Input: part model. Units: mm. Frame: model coordinates. Face numbers are marked on the shaded views. A direction names the side the tool comes from. Round coordinates to 2 decimals unless told otherwise and drop trailing zeros. Loops run counter-clockwise (first coordinate to the right, second up) from the corner with the lowest first, then second, coordinate; pieces in that order, holes last. Notation, with made-up numbers: (-39, 39) - (-34, 39) arc R7 ccw to (-34, 49) - close; hole circle Ø4 at (-32.5, 80). An arc over 180 degrees is marked (long way). Use CSV: the item, a comma, the result in double quotes. Start each with the question number.
1. Cut plane A-A (z = -180). Return loops of the section in (x, y).
2. Cut plane C-C (y = 15). Return loops of the section in (x, z).
3. Cut plane D-D (z = -88.5). Return loops of the section in (x, y).
4. Pull-direction query (Y, two-part tool) for the marked faces 1, 2 and 3; classes: +Y half, -Y half, draft (parallel to the pull), parting line (faces both ways), or undercut.
5. Cut plane B-B (x = 50). Return loops of the section in (y, z).
6. Access query for the marked faces 4, 5 and 6. Directions: +Z, -Z, +X, -X, +Y, -Y. A direction counts if a zero-diameter tool reaches every point of the face in a straight line with its end or side. Return the directions, or none.
7. Material intervals for probe 1 along Y at (x, z) = (50, -14); probe 2 along Z at (x, y) = (51.5, 54); probe 3 along X at (y, z) = (25, -23.5), sorted ascending. Write a range as from..to.
8. Pin query (flat end, axial travel): P1, Ø1.5, axis at x = 54, z = -33, coming from the -Y side; P2, Ø4, axis at x = 15, z = -143.5, coming from the +Y side; P3, Ø6, axis at x = 64, z = -27.5, coming from the +Y side (3 decimals). Return the tip coordinate at first contact, or that it passes through.
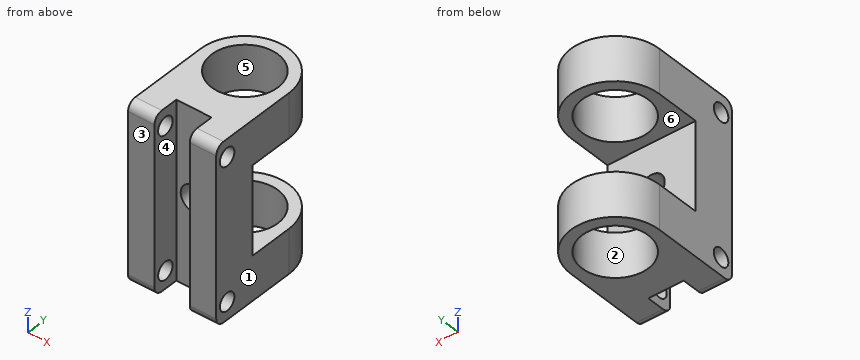
```python
from build123d import *

# Parameters (mm, degrees)
BOSS_EXTRUDE1_DEPTH = 200
SKETCH2_R           = 37.5
SKETCH2_W           = 40
SKETCH2_H           = 30
CUT_EXTRUDE1_DEPTH  = 200
SKETCH3_R           = 10
SKETCH3_W           = 100
SKETCH3_H           = 100
CUT_EXTRUDE2_DEPTH  = 200
SKETCH4_R           = 15
CUT_EXTRUDE3_DEPTH  = 200
FILLET1_R           = 10


with BuildPart() as part:
    # Sketch1 → Boss-Extrude1 (new body)
    with BuildSketch(Plane.XY):
        with BuildLine():
            Line((0, 0), (100, 0))
            Line((100, 0), (100, 100))
            ThreePointArc((100, 100), (50, 150), (0, 100))
            Line((0, 100), (0, 0))
        make_face()
    extrude(amount=-BOSS_EXTRUDE1_DEPTH)

    # Sketch2 → Cut-Extrude1 (cut)
    with BuildSketch(Plane.XY):
        with Locations((50, 100)):
            Circle(SKETCH2_R)
        with Locations((50, 15)):
            Rectangle(SKETCH2_W, SKETCH2_H)
    extrude(amount=-CUT_EXTRUDE1_DEPTH, mode=Mode.SUBTRACT)

    # Sketch3 → Cut-Extrude2 (cut)
    with BuildSketch(Plane(origin=(100, 0, 0), x_dir=(0, 0, -1), z_dir=(1, 0, 0))):
        with Locations((20, 15)):
            Circle(SKETCH3_R)
        with Locations((180, 15)):
            Circle(SKETCH3_R)
        with Locations((100, 100)):
            Rectangle(SKETCH3_W, SKETCH3_H)
    extrude(amount=-CUT_EXTRUDE2_DEPTH, mode=Mode.SUBTRACT)

    # Sketch4 → Cut-Extrude3 (cut)
    with BuildSketch(Plane(origin=(0, 50, 0), x_dir=(1, 0, 0), z_dir=(0, 1, 0))):
        with Locations((50, 100)):
            Circle(SKETCH4_R)
    extrude(amount=-CUT_EXTRUDE3_DEPTH, mode=Mode.SUBTRACT)

    # Fillet1
    fillet1_edges = [part.edges().sort_by_distance(p)[0] for p in [
        (85, 0, 0),
        (85, 0, -200),
        (15, 0, 0),
        (15, 0, -200),
    ]]
    fillet(fillet1_edges, radius=FILLET1_R)


solid = part.part
```
Established:
1,outline,"(0, 0) - (30, 0) - (30, 5) - (0, 5) - close; (0, 25) - (30, 25) - (30, 30) - (70, 30) - (70, 25) - (100, 25) - (100, 100) arc R50 ccw to (0, 100) - close; (70, 0) - (100, 0) - (100, 5) - (70, 5) - close; hole circle Ø75 at (50, 100)"
2,outline,"(0, -200) - (30, -200) - (30, -190) - (0, -190) - close; (0, -170) - (30, -170) - (30, -30) - (0, -30) - close; (0, -10) - (30, -10) - (30, 0) - (0, 0) - close; (70, -200) - (100, -200) - (100, -190) - (70, -190) - close; (70, -170) - (100, -170) - (100, -30) - (70, -30) - close; (70, -10) - (100, -10) - (100, 0) - (70, 0) - close"
3,outline,"(0, 0) - (30, 0) - (30, 30) - (40.37, 30) - (40.37, 50) - (0, 50) - close; (59.63, 30) - (70, 30) - (70, 0) - (100, 0) - (100, 50) - (59.63, 50) - close"
4,face 1,"draft"
4,face 2,"undercut"
4,face 3,"-Y half"
5,outline,"(30, -200) - (62.5, -200) - (62.5, -150) - (50, -150) - (50, -115) - (30, -115) - close; (30, -85) - (50, -85) - (50, -50) - (62.5, -50) - (62.5, 0) - (30, 0) - close; (137.5, -200) - (150, -200) - (150, -150) - (137.5, -150) - close; (137.5, -50) - (150, -50) - (150, 0) - (137.5, 0) - close"
6,face 4,"+Z, -Z, -Y"
6,face 5,"+Z, -Z"
6,face 6,"+X, -X, +Y"
7,probe 1,"y = 30..62.5, 137.5..150"
7,probe 2,"z = -200..-150, -50..0"
7,probe 3,"x = 0..30, 70..100"
8,P1,"stops at y = 30"
8,P2,"stops at y = 50"
8,P3,"stops at y = 148.775"
